Model file for the job. Use its own axes, mm. Round coordinates to 2 decimals unless told otherwise and drop trailing zeros. Loops run counter-clockwise (first coordinate to the right, second up) from the corner with the lowest first, then second, coordinate; pieces in that order, holes last. Notation, with made-up numbers: (81, 80.5) -> (93, 80.5) arc R14 ccw to (93, 84.5) -> close; hole circle Ø7 at (77, 78.5). An arc over 180 degrees is marked (long way). Use a Markdown table: item, result.
from build123d import *

# Parameters (mm, degrees)
CYLINDER1639_R     = 1.5
CYLINDER1639_DEPTH = 60
CYLINDER1640_R     = 1.5
CYLINDER1640_DEPTH = 60
CYLINDER1641_R     = 1.5
CYLINDER1641_DEPTH = 60
CYLINDER1638_R     = 1.5
CYLINDER1638_DEPTH = 60
CYLINDER1628_R     = 7
CYLINDER1628_DEPTH = 48
BOX655_W           = 42
BOX655_H           = 20
BOX655_DEPTH       = 1


with BuildPart() as obj1:
    # Cylinder1639 → Cylinder1639 (new body)
    with BuildSketch(Plane(origin=(18, 85, -57), x_dir=(1, 0, 0), z_dir=(0, 0, 1))):
        Circle(CYLINDER1639_R)
    extrude(amount=CYLINDER1639_DEPTH)


with BuildPart() as obj2:
    # Cylinder1640 → Cylinder1640 (new body)
    with BuildSketch(Plane(origin=(-18, 85, -57), x_dir=(1, 0, 0), z_dir=(0, 0, 1))):
        Circle(CYLINDER1640_R)
    extrude(amount=CYLINDER1640_DEPTH)


with BuildPart() as obj3:
    # Cylinder1641 → Cylinder1641 (new body)
    with BuildSketch(Plane(origin=(-18, 95, -57), x_dir=(1, 0, 0), z_dir=(0, 0, 1))):
        Circle(CYLINDER1641_R)
    extrude(amount=CYLINDER1641_DEPTH)


with BuildPart() as compound810:
    # Cylinder1638 → Cylinder1638 (new body)
    with BuildSketch(Plane(origin=(18, 95, -57), x_dir=(1, 0, 0), z_dir=(0, 0, 1))):
        Circle(CYLINDER1638_R)
    extrude(amount=CYLINDER1638_DEPTH)

    # Compound810: union obj1, obj2, obj3
    add(obj1.part)
    add(obj2.part)
    add(obj3.part)


with BuildPart() as obj4:
    # Cylinder1628 → Cylinder1628 (new body)
    with BuildSketch(Plane(origin=(0, 90, -55), x_dir=(1, 0, 0), z_dir=(0, 0, 1))):
        Circle(CYLINDER1628_R)
    extrude(amount=CYLINDER1628_DEPTH)


with BuildPart() as j_max_encoder_washer:
    # Box655 → Box655 (new body)
    with BuildSketch(Plane(origin=(-21, 80, -39), x_dir=(1, 0, 0), z_dir=(0, 0, 1))):
        with Locations((21, 10)):
            Rectangle(BOX655_W, BOX655_H)
    extrude(amount=BOX655_DEPTH)

    # Cut317: cut obj4
    add(obj4.part, mode=Mode.SUBTRACT)

    # Cut322: cut Compound810
    add(compound810.part, mode=Mode.SUBTRACT)


solid = j_max_encoder_washer.part
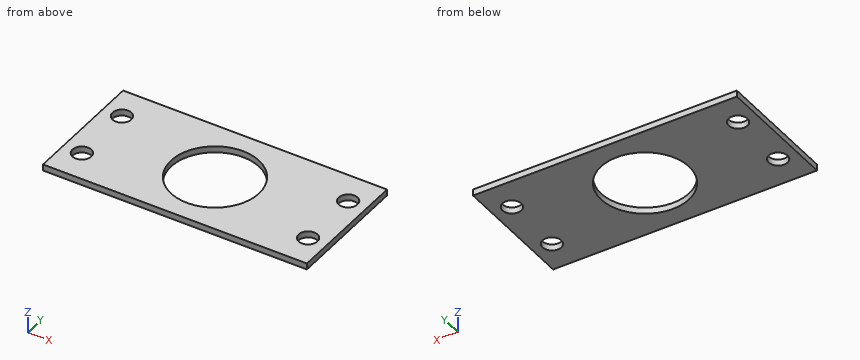
Q1. Band-saw the part on A-A, the plane y = 90. Give the cut face in (x, z).
Results list:
| item | result |
|---|---|
| outline | (-21, -39) -> (-7, -39) -> (-7, -38) -> (-21, -38) -> close; (7, -39) -> (21, -39) -> (21, -38) -> (7, -38) -> close |
Q2. Drill centre lines: L1, parallel to Y at x = -18, z = -38.2; L2, parallel to X at y = 90, z = -38.55; L3, parallel to Y at x = 0, z = -38.55. Where is each one in solid material? Low to high. Write a range as from..to.
Results list:
| item | result |
|---|---|
| L1 | y = 80..83.5, 86.5..93.5, 96.5..100 |
| L2 | x = -21..-7, 7..21 |
| L3 | y = 80..83, 97..100 |
Q3. Band-saw the part on D-D, the plane x = 18. Give the cut face in (y, z).
Results list:
| item | result |
|---|---|
| outline | (80, -39) -> (83.5, -39) -> (83.5, -38) -> (80, -38) -> close; (86.5, -39) -> (93.5, -39) -> (93.5, -38) -> (86.5, -38) -> close; (96.5, -39) -> (100, -39) -> (100, -38) -> (96.5, -38) -> close |
Q4. Band-saw the part on C-C, the plane z = -38.2. Give the cut face in (x, y), plus the area to 3 significant figures.
Results list:
| item | result |
|---|---|
| outline | (-21, 80) -> (21, 80) -> (21, 100) -> (-21, 100) -> close; hole circle Ø3 at (-18, 85); hole circle Ø3 at (-18, 95); hole circle Ø14 at (0, 90); hole circle Ø3 at (18, 85); hole circle Ø3 at (18, 95) |
| area | 658 mm² |
Q5. Flat gauge pin, fed straight in: pin 1 (6 mm diameter, centred on x = 0, y = 93.5, fed in from +Z). Where does the tip first touch, or does it go through?
Results list:
| item | result |
|---|---|
| pin 1 | passes through |
Q6. Band-saw the part on B-B, the plane x = 4. Give the cut face in (y, z), plus the area to 3 significant figures.
Results list:
| item | result |
|---|---|
| outline | (80, -39) -> (84.26, -39) -> (84.26, -38) -> (80, -38) -> close; (95.74, -39) -> (100, -39) -> (100, -38) -> (95.74, -38) -> close |
| area | 8.51 mm² |
